For this review, take the finished solid that the model builds, in its own axes (mm). A direction names the side the tool comes from. Coordinates: 2 decimals unless noted, no trailing zeros. Write each loop counter-clockwise with the first axis right and the second up, starting at its lowest first coordinate (ties: lowest second). Pieces come first, ordered by that corner, then holes.
1) We need section C-C on y = -6. Write out the cut boundary in (x, z), then the cut area to 3 significant figures.
2) We need section A-A on x = 0. Write out the cut boundary in (y, z), then the cut area to 3 significant figures.
3) To check wall thickness, follow line 1 along Y through (x, z) = (-19, 14.5); line 2 along X through (y, z) = (-1, -16); line 3 along X through (y, z) = (-1.75, -16). State the ranges of each line that lie inside material, in increasing order.
4) We need section B-B on z = 0. Write out the cut boundary in (x, y).
5) Insertion check: P1, Ø6, axis at x = 7.5, y = -3.5, coming from the +Z side; P2, Ø8, axis at x = -19, y = 0.5, coming from the -Z side; P3, Ø12, axis at x = 1, z = 22, coming from the +Y side; P4, Ø16, axis at x = -10.5, z = 7, coming from the +Y side. Each pin has a flat end and moves straight along its axis. Give the tip position at first contact, or say it passes through.
6) For faces 1 (the face through (1.08, 2.96, -4.88)), 2 (the face through (0, 6, 0)), list the 3-axis set-ups (+Z, -Z, +X, -X, +Y, -Y) from which the entire face can be reached by the end or side of a thin tool; tool diameter is ignored.
from build123d import *

# Parameters (mm, degrees)
F0_R     = 30
F1_DEPTH = 10
F2_R     = 3
F3_R     = 5
F4_DEPTH = 6


with BuildPart() as f1:
    # F0 (on Front) → F1 (new body)
    with BuildSketch(Plane.XZ):
        Circle(F0_R)
    extrude(amount=F1_DEPTH)

    # F2
    f2_edges = [f1.edges().sort_by_distance(p)[0] for p in [
        (-30, -10, 0),
        (-30, 0, 0),
    ]]
    fillet(f2_edges, radius=F2_R)

    # F3 (on face) → F4 (join)
    with BuildSketch(Plane(origin=(0, 0, 0), x_dir=(-1, 0, 0), z_dir=(0, 1, 0))):
        Circle(F3_R)
    extrude(amount=F4_DEPTH)


solid = f1.part
Result:
1. outline: circle Ø60 at (0, 0)
1. area: 2,830 mm2
2. outline: (-10, -27) arc R3 ccw to (-7, -30) - (-3, -30) arc R3 ccw to (0, -27) - (0, -5) - (6, -5) - (6, 5) - (0, 5) - (0, 27) arc R3 ccw to (-3, 30) - (-7, 30) arc R3 ccw to (-10, 27) - close
2. area: 652 mm2
3. line 1: y = -10 to 0
3. line 2: x = -24.47 to 24.47
3. line 3: x = -25.05 to 25.05
4. outline: (-30, -7) arc R3 ccw to (-27, -10) - (27, -10) arc R3 ccw to (30, -7) - (30, -3) arc R3 ccw to (27, 0) - (5, 0) - (5, 6) - (-5, 6) - (-5, 0) - (-27, 0) arc R3 ccw to (-30, -3) - close
5. P1: stops at z = 29.66
5. P2: stops at z = -25.26
5. P3: stops at y = 0
5. P4: stops at y = 6
6. face 1: +Y
6. face 2: +Z, -Z, +X, -X, +Y
